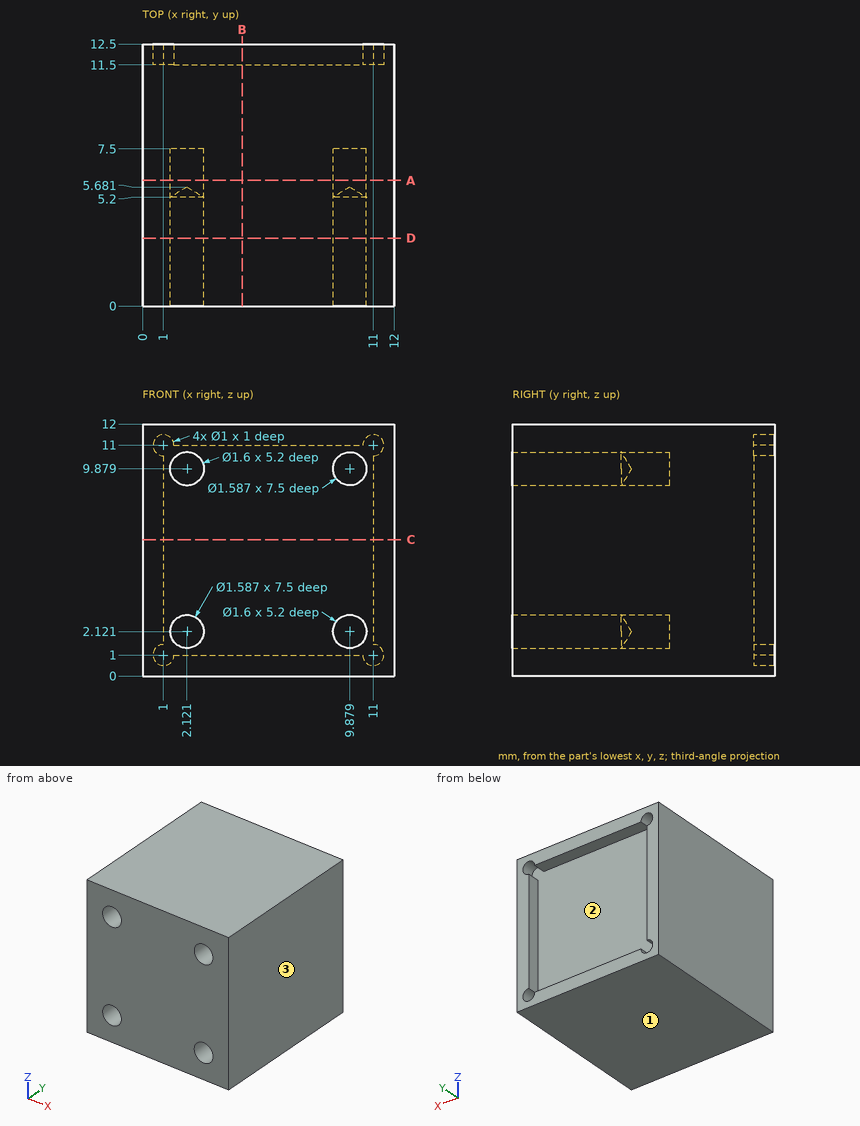
Geometry check sheet. Reference: drawing and pictorial views, mm from the part's lowest x, y, z. Round coordinates to 2 decimals unless told otherwise and drop trailing zeros. Write each loop counter-clockwise with the first axis right and the second up, starting at its lowest first coordinate (ties: lowest second). Pieces come first, ordered by that corner, then holes. Notation, with made-up numbers: (28, 28) -> (39, 28) arc R25 cw to (39, 57) -> close; hole circle Ø7 at (-1, 79.5). An arc over 180 degrees is marked (long way). Answer as CSV lines item,"result". Start each with the question number.
1) Section check B-B on x = 4.75. Enter the section's corners in (y, z).
2) Go/stop test with flat-tipped pins: P1, Ø0.5, axis at x = 2, z = 2, coming from the -Y side; P2, Ø1.3, axis at x = 2.12, z = 2.12, coming from the +Y side; P3, Ø1.4, axis at x = 2.12, z = 9.88, coming from the -Y side. Record where each tip stops, or that it passes through.
3) Section check D-D on y = 3.25. Enter the section's corners in (x, z) (1 decimal).
4) Section check A-A on y = 6. Enter the section's corners in (x, z) (1 decimal), and give its area (3 significant figures).
5) Section check C-C on z = 6.5. Enter the section's corners in (x, y), and give its area (3 significant figures).
6) Material ranges on line 1 (X direction, y = 11.75, z = 1.75); line 2 (Z direction, x = 2, y = 1) (1 decimal); line 3 (Y direction, x = 8, z = 2.5), recorded low to high. Write a range as from..to.
7) Release check for a two-part mould opening along X. For the marked faces 1, 2 and 3 record: pulls with the +X half, pulls with the -X half, needs draft (parallel to the pull), parting line crosses it, or undercut.
Found:
1,outline,"(0, 0) -> (12.5, 0) -> (12.5, 1) -> (11.5, 1) -> (11.5, 11) -> (12.5, 11) -> (12.5, 12) -> (0, 12) -> close"
2,P1,"stops at y = 7.5"
2,P2,"stops at y = 11.5"
2,P3,"stops at y = 5.26"
3,outline,"(0, 0) -> (12, 0) -> (12, 12) -> (0, 12) -> close; hole circle Ø1.6 at (2.1, 2.1); hole circle Ø1.6 at (2.1, 9.9); hole circle Ø1.6 at (9.9, 2.1); hole circle Ø1.6 at (9.9, 9.9)"
4,outline,"(0, 0) -> (12, 0) -> (12, 12) -> (0, 12) -> close; hole circle Ø1.6 at (2.1, 2.1); hole circle Ø1.6 at (9.9, 9.9)"
4,area,"140 mm^2"
5,outline,"(0, 0) -> (12, 0) -> (12, 12.5) -> (11, 12.5) -> (11, 11.5) -> (1, 11.5) -> (1, 12.5) -> (0, 12.5) -> close"
5,area,"140 mm^2"
6,line 1,"x = 0..1, 11..12"
6,line 2,"z = 0..1.3, 2.9..9.1, 10.7..12"
6,line 3,"y = 0..11.5"
7,face 1,"needs draft"
7,face 2,"undercut"
7,face 3,"pulls with the +X half"
